Can you work these out from the drawing? Everything is in mm from the part's minimum corner. A direction names the side the tool comes from. Coordinates: 2 decimals unless noted, no trailing zeros. Write each loop counter-clockwise with the first axis right and the second up, starting at its lowest first coordinate (ties: lowest second). Pieces come first, ordered by that corner, then holes. Notation, with made-up numbers: M 13.5,89 L 68.5,89 A23 cw 68.5,125 Z; hole C 85.5,75 d6. An arc over 180 degrees is marked long. Use one line per item in the form item = value. Start each with the question number.
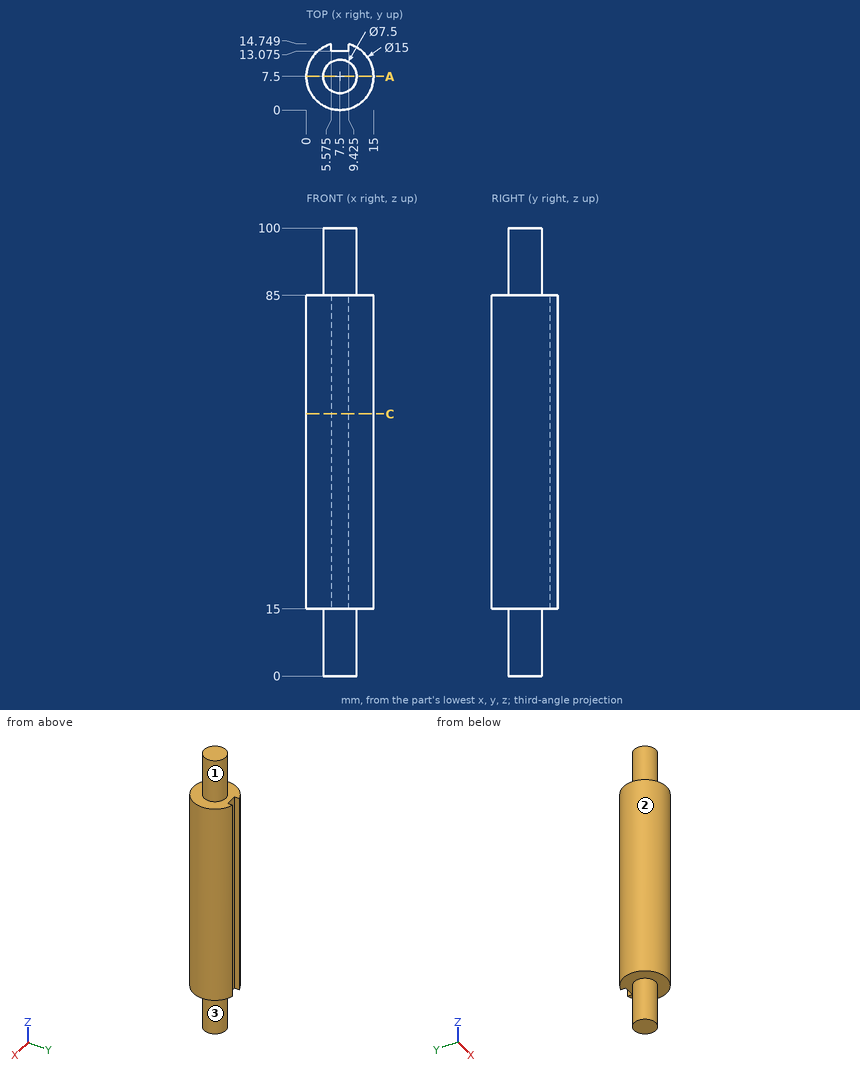
1) Suppose I cut it at C-C on z = 58.5. Please give me the cut outline in (x, y) (1 decimal).
2) Suppose I cut it at A-A on y = 7.5. Please give me the cut outline in (x, z), and give its area (4 significant figures).
3) Please list where these lines run through material, in increasing order: line 1 (Z direction, x = 6.5, y = 3); line 2 (X direction, y = 14.25, z = 34) (1 decimal); line 3 (Y direction, x = 7.75, z = 75) (1 decimal).
4) Will these pins go through, and if not, where does the flat tip stop? pin 1 Ø8 at (y, z) = (9.5, 24) entering from -X; pin 2 Ø1.5 at (x, z) = (2, 23.5) entering from -Y; pin 3 Ø3 at (y, z) = (3.5, 15.5) entering from +X; pin 4 Ø1.3 at (y, z) = (14, 40) entering from +X.
5) Which directions (+Z, -Z, +X, -X, +Y, -Y) give clear straight access to the entire face, cutting with the end or side of a thin tool? Please do the marked faces 1, 2 and 3.
Computed values:
q1.outline = M 5.6,13.1 L 5.6,14.7 A7.5 ccw long 9.4,14.7 L 9.4,13.1 Z
q2.outline = M 0,15 L 3.75,15 L 3.75,0 L 11.25,0 L 11.25,15 L 15,15 L 15,85 L 11.25,85 L 11.25,100 L 3.75,100 L 3.75,85 L 0,85 Z
q2.area = 1,275 mm²
q3.line_1 = 15 to 85
q3.line_2 = 4.2 to 5.6, 9.4 to 10.8
q3.line_3 = 0 to 13.1
q4.pin_1 = 0
q4.pin_2 = 1.7
q4.pin_3 = 14.57
q4.pin_4 = 12.19
q5.face_1 = +Z
q5.face_2 = +Z, -Z
q5.face_3 = -Z
